from build123d import *

# Parameters (mm, degrees)
SKETCH_1_W          = 25
SKETCH_1_H          = 25
EXTRUDE_1_DEPTH     = 7.5
CUT_EXTRUDE_START   = -7.5
CUT_EXTRUDE_3_DEPTH = 7.5
SKETCH_4_R          = 2.2
CUT_EXTRUDE_4_DEPTH = 20.20286437
CUT_EXTRUDE_5_DEPTH = 2
CHAMFER_1_SIZE      = 4
CHAMFER_2_SIZE      = 5
FILLET_3_R          = 2


with BuildPart() as part:
    # ｽｹｯﾁ1 → ﾎﾞｽ - 押し出し1 (new, symmetric)
    with BuildSketch(Plane(origin=(0, 0, 0), x_dir=(1, 0, 0), z_dir=(0, 1, 0))):
        Rectangle(SKETCH_1_W, SKETCH_1_H)
    extrude(amount=EXTRUDE_1_DEPTH, both=True)

    # ｽｹｯﾁ2 → ｶｯﾄ - 押し出し3 (cut)
    with BuildSketch(Plane(origin=(0, 7.5, 0), x_dir=(1, 0, 0), z_dir=(0, 1, 0)).offset(CUT_EXTRUDE_START)):
        with BuildLine():
            Line((12.5, 0), (5, 0))
            ThreePointArc((5, 0), (-3.535533906, 3.535533906), (0, -5))
            Line((0, -5), (0, -12.5))
            Line((0, -12.5), (12.5, -12.5))
            Line((12.5, -12.5), (12.5, 0))
        make_face()
    extrude(amount=CUT_EXTRUDE_3_DEPTH, mode=Mode.SUBTRACT)

    # ｽｹｯﾁ4 → ｶｯﾄ - 押し出し4 (cut, through all)
    with BuildSketch(Plane(origin=(0, 0, 0), x_dir=(1, 0, 0), z_dir=(0, 1, 0))):
        with Locations(Location((0, 0, 0), (0, 0, 270))):
            Circle(SKETCH_4_R)
    extrude(amount=-CUT_EXTRUDE_4_DEPTH, mode=Mode.SUBTRACT)

    # ｽｹｯﾁ5 → ｶｯﾄ - 押し出し5 (cut)
    with BuildSketch(Plane.XZ.offset(7.5)):
        Polygon((-12.5, -1.681266248), (1.681266248, 12.5), (12.5, 12.5), (12.5, 1.681266248), (-1.681266248, -12.5), (-12.5, -12.5), align=None)
    extrude(amount=-CUT_EXTRUDE_5_DEPTH, mode=Mode.SUBTRACT)

    # 面取り1
    chamfer_1_edges = [part.edges().sort_by_distance(p)[0] for p in [
        (-12.5, 0, 12.5),
        (-12.5, 1, -12.5),
        (12.5, 0, -12.5),
    ]]
    chamfer(chamfer_1_edges, length=CHAMFER_1_SIZE)

    # 面取り2
    chamfer_2_edges = [part.edges().sort_by_distance(p)[0] for p in [
        (-10.5, 7.5, -10.5),
    ]]
    chamfer(chamfer_2_edges, length=CHAMFER_2_SIZE)

    # ﾌｨﾚｯﾄ3
    fillet_3_edges = [part.edges().sort_by_distance(p)[0] for p in [
        (12.5, 3.75, 0),
        (0, 3.75, 12.5),
        (0, 3.75, 5),
        (5, 3.75, 0),
    ]]
    fillet(fillet_3_edges, radius=FILLET_3_R)


solid = part.part
Geometry: final body of the model. Coordinates: model frame, mm. A direction names the side the tool comes from. Give positions to 0.01 mm unless a question says otherwise; leave off trailing zeros. Write each loop counter-clockwise with the first axis right and the second up, starting at its lowest first coordinate (ties: lowest second). Pieces come first, ordered by that corner, then holes.
(1) Access query for faces 5 (the cylindrical face through (5.499, 3.802, -0.407)), 6 (the flat face through (5.51, -6.51, -5.31)), 7 (the cylindrical face through (-0.6, 3.8, 11.93)), 8 (the flat face through (0, 0, -12.5)). Directions: +Z, -Z, +X, -X, +Y, -Y. A direction counts if a zero-diameter tool reaches every point of the face in a straight line with its end or side. Return the directions, or none.
(2) Cut plane D-D, the plane z = -4. Return loops of the section in (x, y).
(3) Cut plane C-C, the plane x = -9. Return loops of the section in (y, z), then the cut area to 3 significant figures.
(4) Cut plane A-A, the plane y = -3. Return loops of the section in (x, z), then the cut area to 3 significant figures.
(5) First-contact query: P1, Ø6, axis at x = 0, z = 0, coming from the -Y side; P2, Ø3, axis at y = 3, z = 8, coming from the +X side; P3, Ø3, axis at y = 5, z = -8.5, coming from the -X side. Flat tips, straight axial feed; report the tip coordinate or a pass-through.
(6) Ray query, line 1 (X direction, y = -1.4, z = 0); line 2 (Y direction, x = 6, z = 3.25); line 3 (X direction, y = 1.5, z = 8). Return the intervals inside material, ascending.
(7) Mould query, pull axis X, two halves, no side actions, for faces 1 (the flat face through (7, -7.5, -7)), 2 (the cylindrical face through (-0.386, 3.802, 5.527)), 3 (the cylindrical face through (-3, 4, -4)), 4 (the flat face through (-10, 0, 11)). Classes: released by +X, released by -X, zero draft, split by the parting line, or undercut.
(8) Cut plane B-B, the plane y = 2. Return loops of the section in (x, z).
Values follow:
1. face 5: +Z, +Y
1. face 6: -Y
1. face 7: +Z, +X, +Y
1. face 8: -Z, +X, -X, +Y, -Y
2. outline: (-12.5, -5.5) - (6.82, -5.5) - (6.82, -7.5) - (12.5, -7.5) - (12.5, 7.5) - (3, 7.5) - (3, 0) - (-3, 0) - (-3, 7.5) - (-9.93, 7.5) - (-12.5, 5.68) - close
3. outline: (-7.5, 1.82) - (-5.5, 1.82) - (-5.5, -12) - (2.5, -12) - (7.5, -4.93) - (7.5, 12) - (-7.5, 12) - close
3. area: 315 mm2
4. outline: (-12.5, -8.5) - (-8.5, -12.5) - (8.5, -12.5) - (12.5, -8.5) - (12.5, 12.5) - (-8.5, 12.5) - (-12.5, 8.5) - close; hole circle Ø4.4 at (0, 0)
4. area: 586 mm2
5. P1: stops at y = -5.5
5. P2: stops at x = 0
5. P3: stops at x = -11.56
6. line 1: x = -12.5 to -2.2, 2.2 to 12.5
6. line 2: y = -5.5 to 0
6. line 3: x = -12.5 to 0
7. face 1: zero draft
7. face 2: released by +X
7. face 3: undercut
7. face 4: released by -X
8. outline: (-12.5, -8.5) - (-8.5, -12.5) - (8.5, -12.5) - (12.5, -8.5) - (12.5, -2) arc R2 ccw to (10.5, 0) - (6.71, 0) arc R2 ccw to (4.79, -1.43) arc R5 cw (long way) to (-1.43, 4.79) arc R2 ccw to (0, 6.71) - (0, 10.5) arc R2 ccw to (-2, 12.5) - (-8.5, 12.5) - (-12.5, 8.5) - close
